```python
from build123d import *

# Parameters (mm, degrees)
SKETCH1_W           = 56
SKETCH1_H           = 56
SKETCH1_W_2         = 50
SKETCH1_H_2         = 50
BOSS_EXTRUDE1_DEPTH = 1
SKETCH1_3_W         = 56
SKETCH1_3_H         = 56
SKETCH1_3_W_2       = 50
SKETCH1_3_H_2       = 50
BOSS_EXTRUDE2_DEPTH = 2
SKETCH2_W           = 8
SKETCH2_H           = 19.436412374
CUT_EXTRUDE1_DEPTH  = 1


with BuildPart() as part:
    # Sketch1 → Boss-Extrude1 (new body)
    with BuildSketch(Plane(origin=(0, 0, 0), x_dir=(1, 0, 0), z_dir=(0, 1, 0))):
        Rectangle(SKETCH1_W, SKETCH1_H)
        Rectangle(SKETCH1_W_2, SKETCH1_H_2, mode=Mode.SUBTRACT)
        Rectangle(SKETCH1_W_2, SKETCH1_H_2)
    extrude(amount=BOSS_EXTRUDE1_DEPTH)

    # Sketch1_3 → Boss-Extrude2 (add)
    with BuildSketch(Plane(origin=(0, 0, 0), x_dir=(1, 0, 0), z_dir=(0, 1, 0))):
        Rectangle(SKETCH1_3_W, SKETCH1_3_H)
        Rectangle(SKETCH1_3_W_2, SKETCH1_3_H_2, mode=Mode.SUBTRACT)
    extrude(amount=BOSS_EXTRUDE2_DEPTH)

    # Sketch2 → Cut-Extrude1 (cut)
    with BuildSketch(Plane(origin=(0, 2, 0), x_dir=(1, 0, 0), z_dir=(0, 1, 0))):
        with Locations((0, 31.957312715)):
            Rectangle(SKETCH2_W, SKETCH2_H)
    extrude(amount=-CUT_EXTRUDE1_DEPTH, mode=Mode.SUBTRACT)


solid = part.part
```
Source: CAD feature listing. Evaluate the final solid. Frame: model axes, mm. Coordinates: 2 decimals unless noted, no trailing zeros. Write each loop counter-clockwise with the first axis right and the second up, starting at its lowest first coordinate (ties: lowest second). Pieces come first, ordered by that corner, then holes. Notation, with made-up numbers: (-20.5, -3.75) -> (26.5, -3.75) arc R24 cw to (26.5, 23.25) -> close; hole circle Ø9 at (48, 10.5). An arc over 180 degrees is marked (long way). Return JSON: item names as keys, results as strings. Group by question number.
1) Mould query, pull axis Z, two halves, no side actions, for faces 1 (the face through (-28, 1, 0)), 2 (the face through (-0.4, 0.8, -28)), 3 (the face through (0, 1, -2)). Classes: +Z half, -Z half, draft (parallel to the pull), parting line (faces both ways), or undercut.
2) Ray query, line 1 along Z through (x, y) = (8, 1.6); line 2 along Y through (x, z) = (-19.5, 17). Return the intervals inside material, ascending.
3) Section query A-A, the plane x = 13. Return loops of the section in (y, z), plus the area to 3 significant figures.
4) Contact query for a flat-ended pin moving along its axis: P1, Ø5, axis at x = 1, z = 15.5, coming from the +Y side. Output: stop coordinate, or through.
5) Section query B-B, the plane z = 18.5. Return loops of the section in (x, y), plus the area to 3 significant figures.
From the geometry:
{
 "1": {"face 1": "draft", "face 2": "-Z half", "face 3": "undercut"},
 "2": {"line 1": "-28 to -25, 25 to 28", "line 2": "0 to 1"},
 "3": {"outline": "(0, -28) -> (2, -28) -> (2, -25) -> (1, -25) -> (1, 25) -> (2, 25) -> (2, 28) -> (0, 28) -> close", "area": "62.0 mm²"},
 "4": {"P1": "y = 1"},
 "5": {"outline": "(-28, 0) -> (28, 0) -> (28, 2) -> (25, 2) -> (25, 1) -> (-25, 1) -> (-25, 2) -> (-28, 2) -> close", "area": "62.0 mm²"}
}
